```python
from build123d import *

# Parameters (mm, degrees)
F0_R     = 20
F0_R_2   = 11
F0_R_3   = 6
F1_DEPTH = 24
F2_R     = 6
F3_DEPTH = 24.001
F4_R     = 20
F4_R_2   = 11
F5_DEPTH = 18
F6_R     = 2.25
F7_DEPTH = 6.001


with BuildPart() as f1:
    # F0 (on Front) → F1 (new body)
    with BuildSketch(Plane.XZ):
        Circle(F0_R)
        Circle(F0_R_2, mode=Mode.SUBTRACT)
        Circle(F0_R_2)
        Circle(F0_R_3, mode=Mode.SUBTRACT)
        Circle(F0_R_3)
    extrude(amount=F1_DEPTH)

    # F2 (on face) → F3 (cut, through all)
    with BuildSketch(Plane(origin=(0, 0, 0), x_dir=(-1, 0, 0), z_dir=(0, 1, 0))):
        Circle(F2_R)
    extrude(amount=-F3_DEPTH, mode=Mode.SUBTRACT)

    # F4 (on face) → F5 (cut)
    with BuildSketch(Plane(origin=(0, 0, 0), x_dir=(-1, 0, 0), z_dir=(0, 1, 0))):
        Circle(F4_R)
        Circle(F4_R_2, mode=Mode.SUBTRACT)
    extrude(amount=-F5_DEPTH, mode=Mode.SUBTRACT)

    # F6 (on face) → F7 (cut, through all)
    with BuildSketch(Plane(origin=(0, -18, 0), x_dir=(-1, 0, 0), z_dir=(0, 1, 0))):
        with Locations((-16, 0)):
            Circle(F6_R)
        with Locations((0, -16)):
            Circle(F6_R)
        with Locations((16, 0)):
            Circle(F6_R)
        with Locations((0, 16)):
            Circle(F6_R)
    extrude(amount=-F7_DEPTH, mode=Mode.SUBTRACT)


solid = f1.part
```
CAD build for the part. Positions are in the model's coordinates, mm. A direction names the side the tool comes from. Round coordinates to 2 decimals unless told otherwise and drop trailing zeros. Order: outer loops, then holes, each group sorted by start corner. A loop starts at its lowest first (then second) coordinate and runs counter-clockwise, first axis right, second up. Notation, with made-up numbers: (15, 22) - (70, 22) arc R23 cw to (70, 30) - close; hole circle Ø5 at (-2, -10.5). An arc over 180 degrees is marked (long way). Use CSV: the item, a comma, the result in double quotes. Start each with the question number.
1) Pin check, flat tips, straight feed: pin 1 Ø6 at (x, y) = (2, -21.5) entering from +Z; pin 2 Ø12 at (y, z) = (-3.5, 8.5) entering from -X; pin 3 Ø3 at (y, z) = (-20, -9) entering from -X. Stop position of each tip, or through.
2) Saw through at B-B (x = 0). List the corners of the cut face in (y, z), and give its area (3 significant figures).
3) Saw through at C-C (z = -1.5). List the corners of the cut face in (x, y), and give its area (3 significant figures).
4) Saw through at A-A (x = 16). List the corners of the cut face in (y, z).
5) Tool access for faces 4 (the flat face through (-9, -18, -9)), 5 (the cylindrical face through (-18.146, -20.958, 0.676)): list every direction of +Z, -Z, +X, -X, +Y, -Y with a clear straight run to the whole face (end or side of a thin tool).
6) Two-plate mould, pull along X, no slides. Class faces 1 (the cylindrical face through (13.854, -20.958, 0.676)), 2 (the cylindrical face through (2.38, -8.87, -10.74)), 3 (the flat face through (5, 0, -5)): pulls with the +X half, pulls with the -X half, needs draft (parallel to the pull), parting line crosses it, or undercut.
7) Saw through at D-D (z = 16). List the corners of the cut face in (x, y), and give its area (3 significant figures).
8) Wall check: L1, parallel to Z at x = 0, y = -21.35; L2, parallel to Z at x = 0, y = -13.75; L3, parallel to Y at x = -14, z = -13.5. Give the ranges that are in metal, low to high. Write a range as [from, to].
Values follow:
1,pin 1,"stops at z = 20"
1,pin 2,"stops at x = -10.71"
1,pin 3,"stops at x = -18.54"
2,outline,"(-24, -20) - (-18, -20) - (-18, -18.25) - (-24, -18.25) - close; (-24, -13.75) - (-18, -13.75) - (-18, -11) - (0, -11) - (0, -6) - (-24, -6) - close; (-24, 6) - (0, 6) - (0, 11) - (-18, 11) - (-18, 13.75) - (-24, 13.75) - close; (-24, 18.25) - (-18, 18.25) - (-18, 20) - (-24, 20) - close"
2,area,"294 mm2"
3,outline,"(-19.94, -24) - (-17.68, -24) - (-17.68, -18) - (-19.94, -18) - close; (-14.32, -24) - (-5.81, -24) - (-5.81, 0) - (-10.9, 0) - (-10.9, -18) - (-14.32, -18) - close; (5.81, -24) - (14.32, -24) - (14.32, -18) - (10.9, -18) - (10.9, 0) - (5.81, 0) - close; (17.68, -24) - (19.94, -24) - (19.94, -18) - (17.68, -18) - close"
3,area,"313 mm2"
4,outline,"(-24, -12) - (-18, -12) - (-18, -2.25) - (-24, -2.25) - close; (-24, 2.25) - (-18, 2.25) - (-18, 12) - (-24, 12) - close"
5,face 4,"+Y"
5,face 5,"+Y, -Y"
6,face 1,"undercut"
6,face 2,"parting line crosses it"
6,face 3,"needs draft"
7,outline,"(-12, -24) - (-2.25, -24) - (-2.25, -18) - (-12, -18) - close; (2.25, -24) - (12, -24) - (12, -18) - (2.25, -18) - close"
7,area,"117 mm2"
8,L1,"z = [-20, -18.25], [-13.75, -6], [6, 13.75], [18.25, 20]"
8,L2,"z = [-11, -6], [6, 11]"
8,L3,"y = [-24, -18]"
